from build123d import *

# Parameters (mm, degrees)
SKETCH1_W             = 12.7
SKETCH1_H             = 10.16
BOSS_EXTRUDE1_DEPTH   = 7.62
SKETCH11_W            = 2.54
SKETCH11_H            = 7.62
CUT_EXTRUDE1_DEPTH    = 27.583545687
F_6_32_TAPPED_HOLE1_D = 2.7051


with BuildPart() as part:
    # Sketch1 → Boss-Extrude1 (new body)
    with BuildSketch(Plane(origin=(0, 0, 0), x_dir=(1, 0, 0), z_dir=(0, 1, 0))):
        with Locations((17.003691385, -2.54)):
            Rectangle(SKETCH1_W, SKETCH1_H)
    extrude(amount=BOSS_EXTRUDE1_DEPTH)

    # Sketch11 → Cut-Extrude1 (cut, through all)
    with BuildSketch(Plane.XY.offset(7.62)):
        with Locations((11.923691385, 3.81)):
            Rectangle(SKETCH11_W, SKETCH11_H)
    extrude(amount=-CUT_EXTRUDE1_DEPTH, mode=Mode.SUBTRACT)

    # #6-32 Tapped Hole1 (through all)
    with Locations(Plane.XY.offset(7.62)):
        with Locations((18.273691385, 3.81)):
            Hole(F_6_32_TAPPED_HOLE1_D / 2)


solid = part.part
Geometry: final body of the model. Coordinates: model frame, mm. Round coordinates to 2 decimals unless told otherwise and drop trailing zeros. Loops run counter-clockwise (first coordinate to the right, second up) from the corner with the lowest first, then second, coordinate; pieces in that order, holes last. Notation, with made-up numbers: M -34.75,-5 L -0.75,-5 A17 cw -0.75,17 Z; hole C 82.25,36 d1. An arc over 180 degrees is marked long. Put each result on its own line as item: value. Start each with the question number.
(1) Contact query for a flat-ended pin moving along its axis: pin 1 Ø2.5 at (x, y) = (18.27, 3.81) entering from -Z. Output: stop coordinate, or through.
(2) Section query A-A (y = 3.81). Return loops of the section in (x, z).
(3) Material intervals for line 1 along Y through (x, z) = (18.25, 4); line 2 along X through (y, z) = (5, 2.25); line 3 along Y through (x, z) = (17.25, 5), sorted ascending. Write a range as [from, to].
(4) Draft query along Y for faces 1 (the face through (18, 7.62, 2)), 2 (the face through (23.354, 4, 3)), 3 (the face through (19.625, 3.869, 2.469)). Return one class per face: +Y half, -Y half, draft (parallel to the pull), parting line (faces both ways), or undercut.
(5) Section query C-C (z = 4). Return loops of the section in (x, y), then the cut area to 3 significant figures.
(6) Section query B-B (x = 19.25). Return loops of the section in (y, z).
Findings below:
1. pin 1: passes through
2. outline: M 13.19,-2.54 L 16.92,-2.54 L 16.92,7.62 L 13.19,7.62 Z; M 19.63,-2.54 L 23.35,-2.54 L 23.35,7.62 L 19.63,7.62 Z
3. line 1: y = [0, 2.46], [5.16, 7.62]
3. line 2: x = [13.19, 17.63], [18.92, 23.35]
3. line 3: y = [0, 2.93], [4.69, 7.62]
4. face 1: +Y half
4. face 2: draft
4. face 3: undercut
5. outline: M 13.19,0 L 23.35,0 L 23.35,7.62 L 13.19,7.62 Z; hole C 18.27,3.81 d2.71
5. area: 71.7 mm2
6. outline: M 0,-2.54 L 2.87,-2.54 L 2.87,7.62 L 0,7.62 Z; M 4.75,-2.54 L 7.62,-2.54 L 7.62,7.62 L 4.75,7.62 Z
